Design review of the part built by this model. Coordinates are the model's own, in mm. Coordinates: 2 decimals unless noted, no trailing zeros. Write each loop counter-clockwise with the first axis right and the second up, starting at its lowest first coordinate (ties: lowest second). Pieces come first, ordered by that corner, then holes. Notation, with made-up numbers: (76.5, 34) -> (81.5, 34) arc R9 ccw to (81.5, 47) -> close; hole circle Ø4 at (50, 65). An arc over 180 degrees is marked (long way). Write item = value, one per line. Start each with the question number.
Autodesk Fusion 360 part; units mm, degrees
sketch "Sketch1" plane through (0, 0, 0) normal (0, 0, 1) x (1, 0, 0)
  circle A0 centre (0, 0) radius 31.75
  line L0 (-36.5295, 21.0903) -> (-36.5295, -21.0903)
  line L1 (-36.5295, -21.0903) -> (0, -42.1806)
  line L2 (0, -42.1806) -> (36.5295, -21.0903)
  line L3 (36.5295, -21.0903) -> (36.5295, 21.0903)
  line L4 (36.5295, 21.0903) -> (0, 42.1806)
  line L5 (0, 42.1806) -> (-36.5295, 21.0903)
  line L6 (-2.375, 33.75) -> (2.375, 33.75)
  line L7 (2.375, 33.75) -> (2.375, 38.5)
  line L8 (2.375, 38.5) -> (-2.375, 38.5)
  line L9 (-2.375, 38.5) -> (-2.375, 33.75)
  line L10 (-2.375, 33.75) -> (2.375, 38.5) construction
  line L11 (2.375, 33.75) -> (-2.375, 38.5) construction
  point P0 (0, 36.125)
  point P1 (0, 31.75)
  dimension "d1" = 63.5
  dimension "d2" = 4.75
  dimension "d3" = 2
  dimension "d4" = 2
extrude "Extrude1" add sketch "Sketch1" along normal blind 6 contours L0 L1 L2 L3 L4 L5 | L6 L7 L8 L9
extrude "Extrude2" add sketch "Sketch1" against normal blind 1 contours L0 L1 L2 L3 L4 L5 | L6 L7 L8 L9
extrude "Extrude3" cut sketch "Sketch1" along normal blind 33.02 contours L6 L7 L8 L9
sketch "Sketch2" plane through (0, 0, 6) normal (0, 0, 1) x (1, 0, 0)
  line L0 (-2.375, 38.5) -> (2.375, 38.5)
  line L1 (2.375, 38.5) -> (2.375, 33.75)
  line L2 (2.375, 33.75) -> (-2.375, 33.75)
  line L3 (-2.375, 33.75) -> (-2.375, 38.5)
  circle A0 centre (0, 0) radius 31.75
  line L4 (0, 42.1806) -> (-36.5295, 21.0903)
  line L5 (-36.5295, 21.0903) -> (-36.5295, -21.0903)
  line L6 (-36.5295, -21.0903) -> (0, -42.1806)
  line L7 (0, -42.1806) -> (36.5295, -21.0903)
  line L8 (36.5295, -21.0903) -> (36.5295, 21.0903)
  line L9 (36.5295, 21.0903) -> (0, 42.1806)
  line L10 (-8.9538, 50.7426) -> (10.16, 50.7426)
  line L11 (10.16, 50.7426) -> (10.16, 22.86)
  line L12 (10.16, 22.86) -> (-8.9538, 22.86)
  line L13 (-8.9538, 22.86) -> (-8.9538, 50.7426)
extrude "Extrude4" [suppressed]
chamfer "Chamfer1" distance 0.25 angle 45 4 edges at (-2.375, 36.125, 6) (0, 33.75, 6) (2.375, 36.125, 6) (0, 38.5, 6) measured on face at (34.9363, 0, 6) measured on face at (34.9363, 0, 6) measured on face at (34.9363, 0, 6) measured on face at (34.9363, 0, 6)
sketch "Sketch3" plane through (0, 0, 0) normal (0, 0, 1) x (1, 0, 0)
  line L0 (-2.375, 38.5) -> (-2.375, 33.75)
  line L1 (-2.375, 33.75) -> (2.375, 33.75)
  line L2 (2.375, 33.75) -> (2.375, 38.5)
  line L3 (2.375, 38.5) -> (-2.375, 38.5)
  line L4 (2.375, 38.5) -> (-2.375, 33.75)
  point P0 (0, 36.125)
pattern_circular "C-Pattern1" count 6 over 360 about axis through (0, 0, 1.75) along (0, 0, 1) of "Extrude3", "Chamfer1"
(1) For pin 1 Ø1.9 at (x, y) = (-30.5, -18) entering from +Z; pin 2 Ø2.5 at (y, z) = (-37, 3) entering from +X; pin 3 Ø1.5 at (x, z) = (-29, 2.5) entering from +Y, all flat-tipped, find the tip position at first contact; note any pin that passes through.
(2) Mouldability with a two-part tool opening along X and no side actions: class faces 1 (the face through (8, -31, -1)), 2 (the face through (31, 18, 0)) as pulls with the +X half, pulls with the -X half, needs draft (parallel to the pull), parting line crosses it, or undercut.
(3) Take a section at C-C, the plane x = 12.5. State the section outline as (y, z) points.
(4) Take a section at A-A, the plane y = 0. State the section outline as (x, z) points.
(5) Take a section at B-B, the plane z = 2. Count the separate pieces of the cut face and the enclosed holes in it, then the cut area to 3 significant figures.
(6) For line 1 (Y direction, x = 0, z = 1.25); line 2 (X direction, y = 15.5, z = 0.5); line 3 (Y direction, x = 26, z = 3.75), list the stretches that pass through material, from the lowest coordinate up.
Report:
q1.pin_1 = 0
q1.pin_2 = 11.14
q1.pin_3 = 25.87
q2.face_1 = needs draft
q2.face_2 = undercut
q3.outline = (-34.96, -1) -> (-29.19, -1) -> (-29.19, 6) -> (-34.96, 6) -> close; (29.19, -1) -> (34.96, -1) -> (34.96, 6) -> (29.19, 6) -> close
q4.outline = (-36.53, -1) -> (-31.75, -1) -> (-31.75, 6) -> (-36.53, 6) -> close; (31.75, -1) -> (36.53, -1) -> (36.53, 6) -> (31.75, 6) -> close
q5.separate_pieces = 1
q5.enclosed_holes = 7
q5.area = 1,320 mm2
q6.line_1 = -42.18 to -38.5, -33.75 to -31.75, 31.75 to 33.75, 38.5 to 42.18
q6.line_2 = -36.53 to -31.6, -30.02 to -27.71, 27.71 to 30.02, 31.6 to 36.53
q6.line_3 = -27.17 to -18.22, 18.22 to 27.17
